from build123d import *

# Parameters (mm, degrees)
F1_DEPTH  = 12
F2_W      = 200
F2_H      = 20
F3_DEPTH  = 5
F4_W      = 155
F4_H      = 20
F5_DEPTH  = 5
F6_R      = 2.5
F7_DEPTH  = 25
F9_DEPTH  = 5
F10_W     = 195
F10_H     = 30
F10_W_2   = 30
F10_H_2   = 145
F11_DEPTH = 25
F12_W     = 145
F12_H     = 16
F13_DEPTH = 195.0010001


with BuildPart() as f1:
    # F0 (on Top) → F1 (new body)
    with BuildSketch(Plane.XY):
        with BuildLine():
            add(Edge.make_bspline(
                [(-176, 0), (-176, -130), (0, -130)],
                knots=[3.1415926536, 3.1415926536, 3.1415926536, 4.7123889804, 4.7123889804, 4.7123889804], degree=2, weights=[1, 0.7071067812, 1]))
            Line((-176, 0), (-176, -130))
            Line((-176, -130), (0, -130))
        make_face()
        Polygon((-176, -130), (-176, 0), (-200, 0), (-200, -150), (0, -150), (0, -130), align=None)
    extrude(amount=F1_DEPTH)

    # F2 (on face) → F3 (join)
    with BuildSketch(Plane.XZ.offset(150)):
        with Locations((-100, 6)):
            Rectangle(F2_W, F2_H)
    extrude(amount=F3_DEPTH)

    # F4 (on face) → F5 (join)
    with BuildSketch(Plane(origin=(-200, 0, 0), x_dir=(0, -1, 0), z_dir=(-1, 0, 0))):
        with Locations((77.5, 6)):
            Rectangle(F4_W, F4_H)
    extrude(amount=F5_DEPTH)

    # F6 (on face) → F7 (join)
    with BuildSketch(Plane(origin=(0, 0, -4), x_dir=(1, 0, 0), z_dir=(0, 0, -1))):
        Polygon((0, 155), (0, 175), (-225, 175), (-225, 0), (-205, 0), (-205, 155), align=None)
        with Locations((-212.5, 60)):
            Circle(F6_R, mode=Mode.SUBTRACT)
        with Locations((-212.5, 115)):
            Circle(F6_R, mode=Mode.SUBTRACT)
        with Locations((-165, 162.5)):
            Circle(F6_R, mode=Mode.SUBTRACT)
        with Locations((-60, 162.5)):
            Circle(F6_R, mode=Mode.SUBTRACT)
    extrude(amount=-F7_DEPTH)

    # F8 (on face) → F9 (join)
    with BuildSketch(Plane.XY.offset(16)):
        Polygon((-190, 0), (-205, 0), (-205, -155), (0, -155), (0, -140), (-190, -140), align=None)
    extrude(amount=F9_DEPTH)

    # F10 (on Top) → F11 (cut, symmetric)
    with BuildSketch(Plane.XY):
        with Locations((-127.5, -15)):
            Rectangle(F10_W, F10_H)
        with Locations((-15, -15)):
            Rectangle(F10_W_2, F10_H)
        with Locations((-15, -102.5)):
            Rectangle(F10_W_2, F10_H_2)
    extrude(amount=F11_DEPTH, both=True, mode=Mode.SUBTRACT)

    # F12 (on face) → F13 (cut, through all)
    with BuildSketch(Plane.YZ.offset(-30)):
        with Locations((-102.5, 4)):
            Rectangle(F12_W, F12_H)
    extrude(amount=-F13_DEPTH, mode=Mode.SUBTRACT)


solid = f1.part
CAD build for the part. Positions are in the model's coordinates, mm. A direction names the side the tool comes from. Give positions to 0.01 mm unless a question says otherwise; leave off trailing zeros. Write each loop counter-clockwise with the first axis right and the second up, starting at its lowest first coordinate (ties: lowest second). Pieces come first, ordered by that corner, then holes. Notation, with made-up numbers: (19, -38) -> (56, -38) arc R8 ccw to (56, -25) -> close; hole circle Ø2 at (-18, 23.5). An arc over 180 degrees is marked (long way). Return JSON: item names as keys, results as strings.
Item 1: Two-plate mould, pull along X, no slides. Class faces 4 (the flat face through (-190, -86, 18)), 5 (the cylindrical face through (-210.115, -60.751, 16.437)), 6 (the flat face through (-126, -175, 16)): +X half, -X half, draft (parallel to the pull), parting line (faces both ways), or undercut.
Answer below:
{"face 4": "+X half", "face 5": "undercut", "face 6": "draft"}
Item 2: Drop flat-ended pins along their axis: pin 1 (2 mm diameter, centred on y = -109.5, z = 13.5, fed in from +X); pin 2 (2.5 mm diameter, centred on y = -74, z = 19.5, fed in from +X); pin 3 (3 mm diameter, centred on x = -89.5, z = 20, fed in from +Y); pin 4 (4 mm diameter, centred on x = -165, y = -162.5, fed in from +Z). Give the stop position or say it passes through.
Answer below:
{"pin 1": "stops at x = -200", "pin 2": "stops at x = -190", "pin 3": "stops at y = -140", "pin 4": "passes through"}
Item 3: Band-saw the part on D-D (x = -60). List the corners of the cut face in (y, z), then the cut area to 3 significant figures.
Answer below:
{"outline": "(-175, 12) -> (-165, 12) -> (-165, 21) -> (-175, 21) -> close; (-160, 12) -> (-150, 12) -> (-150, 16) -> (-140, 16) -> (-140, 21) -> (-160, 21) -> close", "area": "230 mm2"}
Item 4: Drill centre lines: probe 1 along X at (y, z) = (-162.5, 15.25); probe 2 along X at (y, z) = (-115, 18.75); probe 3 along Y at (x, z) = (-212.5, 18.5). Where is each one in solid material? Low to high.
Answer below:
{"probe 1": "x = -225 to -167.5, -162.5 to -62.5, -57.5 to -30", "probe 2": "x = -225 to -215, -210 to -190", "probe 3": "y = -175 to -117.5, -112.5 to -62.5, -57.5 to -30"}
Item 5: Band-saw the part on C-C (z = 14.5). List the corners of the cut face in (x, y), then the cut area to 3 significant figures.
Answer below:
{"outline": "(-225, -175) -> (-30, -175) -> (-30, -150) -> (-200, -150) -> (-200, -30) -> (-225, -30) -> close; hole circle Ø5 at (-212.5, -115); hole circle Ø5 at (-212.5, -60); hole circle Ø5 at (-165, -162.5); hole circle Ø5 at (-60, -162.5)", "area": "7,800 mm2"}
Item 6: Band-saw the part on B-B (x = -212.5). List the corners of the cut face in (y, z).
Answer below:
{"outline": "(-175, 12) -> (-117.5, 12) -> (-117.5, 21) -> (-175, 21) -> close; (-112.5, 12) -> (-62.5, 12) -> (-62.5, 21) -> (-112.5, 21) -> close; (-57.5, 12) -> (-30, 12) -> (-30, 21) -> (-57.5, 21) -> close"}
Item 7: Tool access for faces 1 (the flat face through (-225, -104, 16)), 2 (the flat face through (-109, -140, 18)), 3 (the flat face through (-200, -89, 14)): list every direction of +Z, -Z, +X, -X, +Y, -Y with a clear straight run to the whole face (end or side of a thin tool).
Answer below:
{"face 1": "+Z, -Z, -X, +Y, -Y", "face 2": "+Z, -Z, +X, +Y", "face 3": "-Z, +X, +Y"}
Item 8: Band-saw the part on A-A (y = -115). List the corners of the cut face in (x, z).
Answer below:
{"outline": "(-225, 12) -> (-215, 12) -> (-215, 21) -> (-225, 21) -> close; (-210, 12) -> (-200, 12) -> (-200, 16) -> (-190, 16) -> (-190, 21) -> (-210, 21) -> close"}
